Read the model definition and answer for the solid it produces. Units are mm, in the model's axes. Face numbers are marked on the shaded views. Coordinates: 2 decimals unless noted, no trailing zeros. Loops run counter-clockwise (first coordinate to the right, second up) from the corner with the lowest first, then second, coordinate; pieces in that order, holes last.
Q1. Section A-A (y = 0) is taken. Give the vertices of the cut face in (x, z), then the cut area to 3 significant figures.
Q2. Section B-B (z = 2.65) is taken. Count the separate pieces of the cut face and the enclosed holes in it, then the cut area to 3 significant figures.
Q3. Section D-D (y = 45) is taken. Give the vertices of the cut face in (x, z), then the cut area to 3 significant figures.
Q4. Straight lines are drawn through the part: line 1 (X direction, y = 100, z = 3.1); line 2 (X direction, y = 91.15, z = 2.95); line 3 (X direction, y = 2, z = 1.25). For each, find the intervals that lie inside material, in ascending order.
Q5. Flat-ended cylindrical pins translate along their axes: P1, Ø4.5, axis at x = 0, y = 0, coming from the -Z side; P2, Ø3, axis at y = 16.5, z = 4, coming from the -X side; P3, Ø3, axis at x = 15, z = 3, coming from the +Y side; P4, Ø2.5, axis at y = 84.5, z = 3, coming from the +X side. Find the tip coordinate at first contact, or state that the pin passes through.
Q6. The mould has two halves that part along Z. Classify the marked faces 1 and 2: pulls with the +Z half, pulls with the -Z half, needs draft (parallel to the pull), parting line crosses it, or undercut.
Q7. Section C-C (x = 24) is taken. Give the vertices of the cut face in (y, z), then the cut area to 3 significant figures.
from build123d import *

# Parameters (mm, degrees)
SKETCH1_R           = 1.05
SKETCH1_R_2         = 0.6
SKETCH1_R_3         = 2.5
BOSS_EXTRUDE1_DEPTH = 5


with BuildPart() as part:
    # Sketch1 → Boss-Extrude1 (new body)
    with BuildSketch(Plane.XY):
        with BuildLine():
            Line((-12.5, 120), (12.5, 120))
            Line((12.5, 120), (12.5, 30.310889132))
            ThreePointArc((12.5, 30.310889132), (13.169872981, 27.810889132), (15, 25.980762114))
            ThreePointArc((15, 25.980762114), (0, -30), (-15, 25.980762114))
            ThreePointArc((-15, 25.980762114), (-13.169872981, 27.810889132), (-12.5, 30.310889132))
            Line((-12.5, 30.310889132), (-12.5, 120))
        make_face()
        with Locations((0, 100)):
            Circle(SKETCH1_R, mode=Mode.SUBTRACT)
        with Locations((0, 95.15)):
            Circle(SKETCH1_R_2, mode=Mode.SUBTRACT)
        with Locations((0, 93.15)):
            Circle(SKETCH1_R_2, mode=Mode.SUBTRACT)
        with Locations((0, 91.15)):
            Circle(SKETCH1_R_2, mode=Mode.SUBTRACT)
        with Locations((0, 89.15)):
            Circle(SKETCH1_R_2, mode=Mode.SUBTRACT)
        with Locations((0, 87.15)):
            Circle(SKETCH1_R_2, mode=Mode.SUBTRACT)
        with Locations((0, 85.15)):
            Circle(SKETCH1_R_2, mode=Mode.SUBTRACT)
        with Locations((0, 83.15)):
            Circle(SKETCH1_R_2, mode=Mode.SUBTRACT)
        with Locations((6.45, 100)):
            Circle(SKETCH1_R_2, mode=Mode.SUBTRACT)
        with Locations((4.45, 100)):
            Circle(SKETCH1_R_2, mode=Mode.SUBTRACT)
        with Locations((-4.45, 100)):
            Circle(SKETCH1_R_2, mode=Mode.SUBTRACT)
        with Locations((-6.45, 100)):
            Circle(SKETCH1_R_2, mode=Mode.SUBTRACT)
        with Locations((0, 104.45)):
            Circle(SKETCH1_R_2, mode=Mode.SUBTRACT)
        with Locations((0, 106.45)):
            Circle(SKETCH1_R_2, mode=Mode.SUBTRACT)
        with Locations((0, 108.45)):
            Circle(SKETCH1_R_2, mode=Mode.SUBTRACT)
        with Locations((0, 110.45)):
            Circle(SKETCH1_R_2, mode=Mode.SUBTRACT)
        with Locations((0, 112.45)):
            Circle(SKETCH1_R_2, mode=Mode.SUBTRACT)
        with Locations((0, 114.45)):
            Circle(SKETCH1_R_2, mode=Mode.SUBTRACT)
        Circle(SKETCH1_R_3, mode=Mode.SUBTRACT)
    extrude(amount=BOSS_EXTRUDE1_DEPTH)


solid = part.part
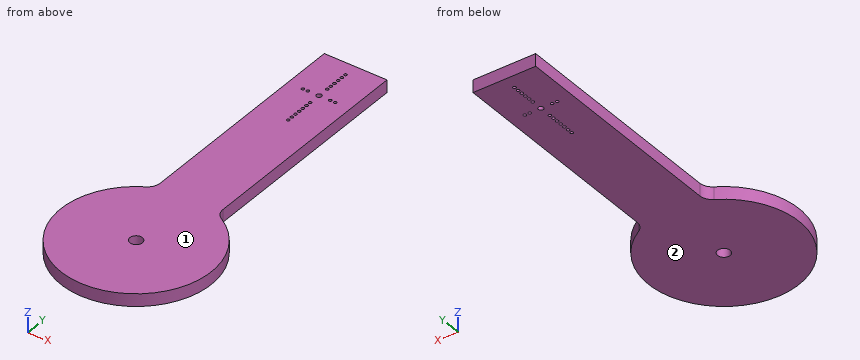
Numbers:
1. outline: (-30, 0) - (-2.5, 0) - (-2.5, 5) - (-30, 5) - close; (2.5, 0) - (30, 0) - (30, 5) - (2.5, 5) - close
1. area: 275 mm2
2. separate pieces: 1
2. enclosed holes: 19
2. area: 5,060 mm2
3. outline: (-12.5, 0) - (12.5, 0) - (12.5, 5) - (-12.5, 5) - close
3. area: 125 mm2
4. line 1: x = -12.5 to -7.05, -5.85 to -5.05, -3.85 to -1.05, 1.05 to 3.85, 5.05 to 5.85, 7.05 to 12.5
4. line 2: x = -12.5 to -0.6, 0.6 to 12.5
4. line 3: x = -29.93 to -1.5, 1.5 to 29.93
5. P1: passes through
5. P2: stops at x = -25.98
5. P3: stops at y = 27.31
5. P4: stops at x = 12.5
6. face 1: pulls with the +Z half
6. face 2: pulls with the -Z half
7. outline: (-18, 0) - (18, 0) - (18, 5) - (-18, 5) - close
7. area: 180 mm2
